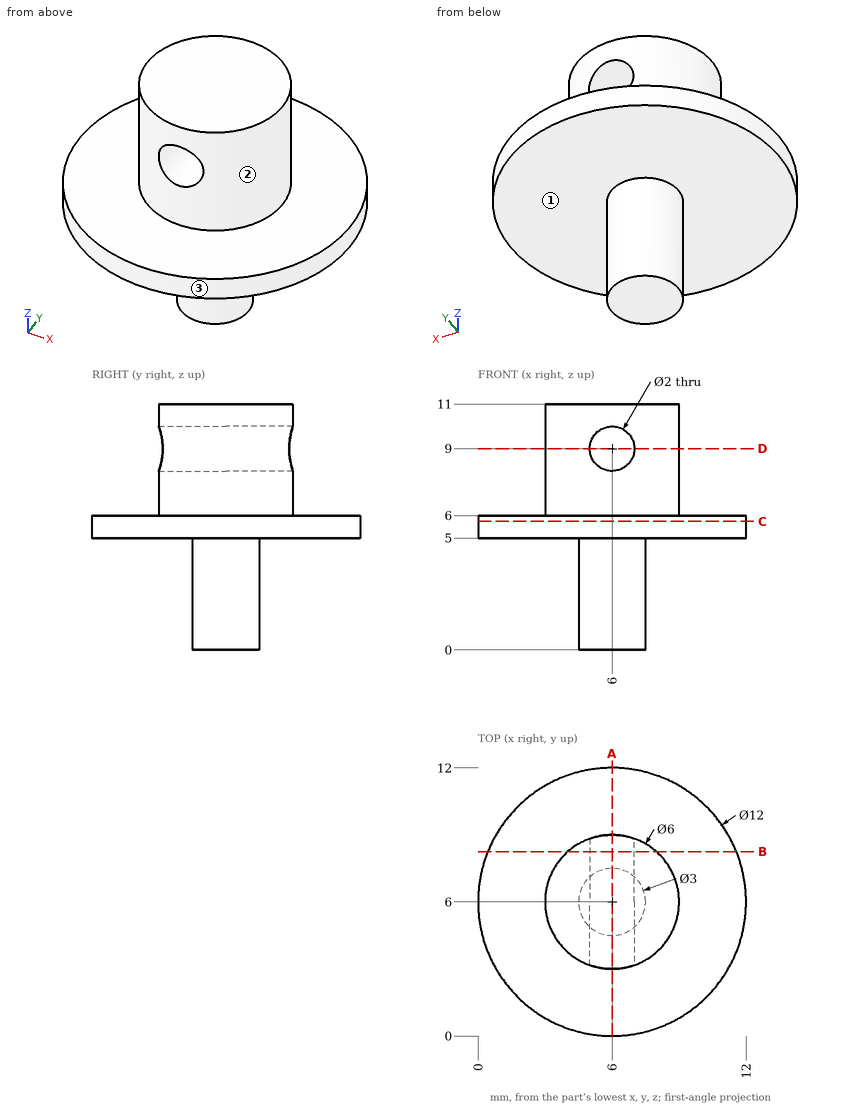
Source: three-view drawing plus pictorial views. Frame: mm from the lowest corner of the part. A direction names the side the tool comes from. Give positions to 0.01 mm unless a question says otherwise; leave off trailing zeros. Order: outer loops, then holes, each group sorted by start corner. A loop starts at its lowest first (then second) coordinate and runs counter-clockwise, first axis right, second up. Notation, with made-up numbers: (79.25, -19.5) -> (123.25, -19.5) arc R10 cw to (123.25, -15.5) -> close; hole circle Ø3 at (-31, 23.5). An arc over 180 degrees is marked (long way). Use a Markdown table: item, result.
Q1. First-contact query: P1, Ø5, axis at x = 2, z = 9.5, coming from the -Y side; P2, Ø2.5, axis at x = 6, z = 9, coming from the +Y side; P3, Ø1.5, axis at x = 4.5, z = 7.5, coming from the +Y side. Flat tips, straight axial feed; report the tip coordinate or a pass-through.
A:
| item | result |
|---|---|
| P1 | y = 3.4 |
| P2 | y = 9 |
| P3 | y = 8.9 |
Q2. Material intervals for line 1 (Z direction, x = 6, y = 8); line 2 (Z direction, x = 6, y = 5); line 3 (Z direction, x = 7.75, y = 4.5), sorted ascending. Write a range as [from, to].
A:
| item | result |
|---|---|
| line 1 | [5, 8], [10, 11] |
| line 2 | [0, 8], [10, 11] |
| line 3 | [5, 11] |
Q3. Access query for the marked faces 1, 2 and 3. Directions: +Z, -Z, +X, -X, +Y, -Y. A direction counts if a zero-diameter tool reaches every point of the face in a straight line with its end or side. Return the directions, or none.
A:
| item | result |
|---|---|
| face 1 | -Z |
| face 2 | +Z |
| face 3 | +Z, -Z |
Q4. Section A-A (x = 6). Return the cut outline in (y, z).
A:
| item | result |
|---|---|
| outline | (0, 5) -> (4.5, 5) -> (4.5, 0) -> (7.5, 0) -> (7.5, 5) -> (12, 5) -> (12, 6) -> (9, 6) -> (9, 8) -> (3, 8) -> (3, 6) -> (0, 6) -> close; (3, 10) -> (9, 10) -> (9, 11) -> (3, 11) -> close |
Q5. Section B-B (y = 8.25). Return the cut outline in (x, z).
A:
| item | result |
|---|---|
| outline | (0.44, 5) -> (11.56, 5) -> (11.56, 6) -> (7.98, 6) -> (7.98, 11) -> (4.02, 11) -> (4.02, 6) -> (0.44, 6) -> close; hole circle Ø2 at (6, 9) |
Q6. Section C-C (z = 5.75). Return the cut outline in (x, y), and give its area (3 significant figures).
A:
| item | result |
|---|---|
| outline | circle Ø12 at (6, 6) |
| area | 113 mm^2 |
Q7. Section D-D (z = 9). Return the cut outline in (x, y).
A:
| item | result |
|---|---|
| outline | (5, 3.17) -> (5, 8.83) arc R3 ccw to start; (7, 3.17) arc R3 ccw to (7, 8.83) -> close |
